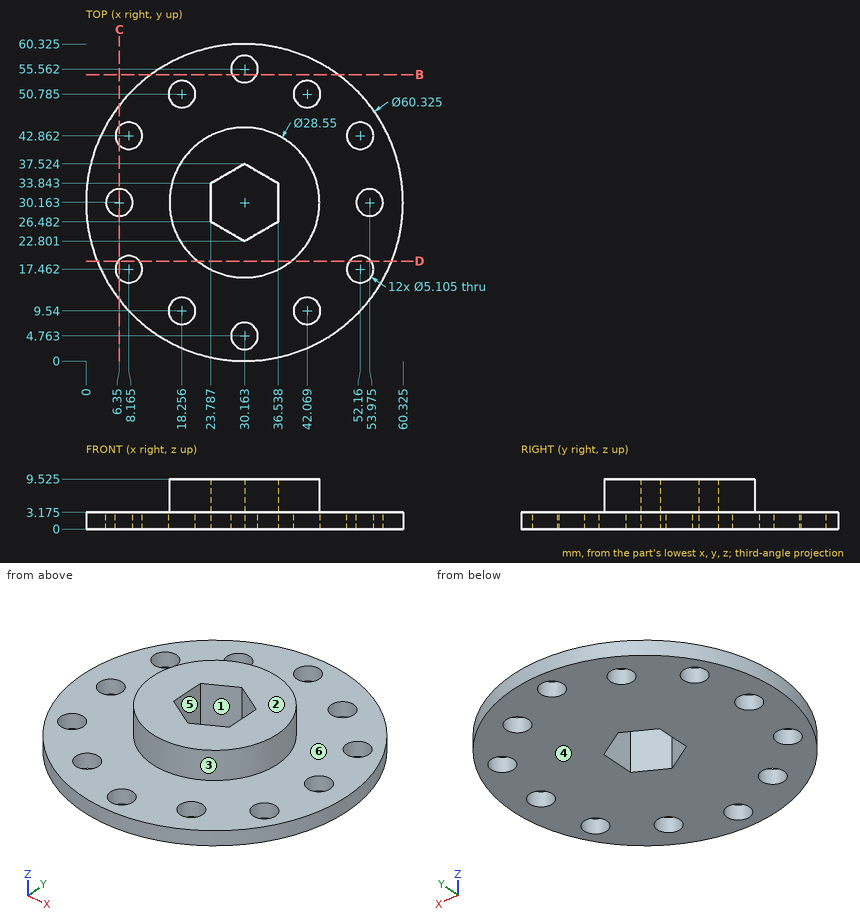
Here's the drawing with two shaded views (mm, measured from the low corner). I have some questions. A direction names the side the tool comes from. Give positions to 0.01 mm unless a question says otherwise; leave off trailing zeros. Loops run counter-clockwise (first coordinate to the right, second up) from the corner with the lowest first, then second, coordinate; pieces in that order, holes last. Notation, with made-up numbers: (-14.5, 33) - (-3.5, 33) arc R27 ccw to (-3.5, 59) - close; hole circle Ø5 at (83.25, 44). An arc over 180 degrees is marked (long way). Return JSON: item names as keys, results as strings.
1. I want a section at D-D on y = 19. Please give me the cut outline in (x, z) (1 decimal), and give its area (3 significant figures).
Output values:
{"outline": "(2.1, 0) - (6.1, 0) - (6.1, 3.2) - (2.1, 3.2) - close; (10.2, 0) - (50.1, 0) - (50.1, 3.2) - (39.1, 3.2) - (39.1, 9.5) - (21.3, 9.5) - (21.3, 3.2) - (10.2, 3.2) - close; (54.2, 0) - (58.2, 0) - (58.2, 3.2) - (54.2, 3.2) - close", "area": "265 mm²"}
2. If I drill on line 1 (Y direction, x = 50, z = 1.25) (1 decimal); line 2 (Z direction, x = 41.5, y = 6) (1 decimal); line 3 (X direction, y = 24, z = 8.5) (1 decimal), over which ranges is the centre line in solid material (lowest first)?
Output values:
{"line 1": "y = 7.4 to 16.1, 18.8 to 41.5, 44.2 to 52.9", "line 2": "z = 0 to 3.2", "line 3": "x = 17.3 to 28.1, 32.2 to 43"}
3. For the marked faces 4, 5 and 6, which set-ups out of +Z, -Z, +X, -X, +Y, -Y let a thin tool reach every point of the face, with its end or its side?
Output values:
{"face 4": "-Z, +X, -X, +Y, -Y", "face 5": "+Z, -Z", "face 6": "+Z"}
4. We'd pull the mould along X, two halves only. Please class the marked faces 1, 2 and 3: +X half, -X half, draft (parallel to the pull), parting line (faces both ways), or undercut.
Output values:
{"face 1": "undercut", "face 2": "draft", "face 3": "parting line"}
5. I want a section at B-B on y = 54.5. Please give me the cut outline in (x, z) (1 decimal).
Output values:
{"outline": "(12.3, 0) - (27.8, 0) - (27.8, 3.2) - (12.3, 3.2) - close; (32.5, 0) - (48, 0) - (48, 3.2) - (32.5, 3.2) - close"}
6. I'm going to push flat-ended pins straight in: pin 1 Ø3 at (x, z) = (28.5, 8) entering from +Y; pin 2 Ø6.5 at (x, y) = (42.07, 9.54) entering from +Z (1 decimal); pin 3 Ø1.5 at (y, z) = (13, 3) entering from -X (1 decimal). Where does each tip first touch, or does it pass through?
Output values:
{"pin 1": "stops at y = 44.44", "pin 2": "stops at z = 3.2", "pin 3": "stops at x = 4.9"}
7. I want a section at C-C on x = 6.35. Give the number of separate pieces and of enclosed holes in the cut face.
Output values:
{"separate pieces": "4", "enclosed holes": "0"}
